Input: part model. Units: mm. Frame: model coordinates. Round coordinates to 2 decimals unless told otherwise and drop trailing zeros. Loops run counter-clockwise (first coordinate to the right, second up) from the corner with the lowest first, then second, coordinate; pieces in that order, holes last.
1) Section A-A, the plane z = -94. Return loops of the section in (x, y), and give its area (3 significant figures).
2) First-contact query: pin 1 (0.9 mm diameter, centred on x = -47, y = 1, fed in from +Z); pin 2 (1.5 mm diameter, centred on x = -105, y = 1, fed in from +Z); pin 3 (0.9 mm diameter, centred on x = -47, y = 1.5, fed in from -Z). Flat tips, straight axial feed; report the tip coordinate or a pass-through.
3) Section B-B, the plane x = -156. Return loops of the section in (y, z), and give its area (3 significant figures).
4) Section C-C, the plane y = 1.85. State how many separate pieces and enclosed holes the cut face has, and give its area (3 significant figures).
5) Section D-D, the plane z = -51. Return loops of the section in (x, y), and give its area (3 significant figures).
6) Ray query, line 1 along Z through (x, y) = (-160, 1.05); line 2 along Z through (x, y) = (-127.5, 1.9); line 3 along X through (y, z) = (2.75, -86.5). Return the intervals inside material, ascending.
Autodesk Inventor part; units mm, degrees
ref_plane "YZ Plane" through (0, 0, 0) normal (1, 0, 0) x (0, 1, 0)
ref_plane "XZ Plane" through (0, 0, 0) normal (0, 1, 0) x (-1, 0, 0)
ref_plane "XY Plane" through (0, 0, 0) normal (0, 0, 1) x (1, 0, 0)
sketch "Sketch1" plane through (0, 0, 0) normal (0, 1, 0) x (-1, 0, 0)
  line L0 (98.8824, -242.8336) -> (78.8824, -242.8336)
  line L1 (98.8824, -237.8336) -> (98.8824, -242.8336)
  line L2 (113.8824, -237.8336) -> (98.8824, -237.8336)
  line L3 (128.8824, -242.8336) -> (113.8824, -242.8336)
  line L4 (128.8824, -242.8336) -> (128.8824, -237.8336)
  line L5 (113.8824, -242.8336) -> (113.8824, -237.8336)
  line L6 (113.8824, 65.1664) -> (113.8824, 62.1664)
  line L7 (98.8824, 62.1664) -> (98.8824, 65.1664)
  line L8 (78.8824, 65.1664) -> (98.8824, 65.1664)
  line L9 (98.8824, 62.1664) -> (113.8824, 62.1664)
  line L10 (113.8824, 65.1664) -> (128.8824, 65.1664)
  line L11 (128.8824, 62.1664) -> (128.8824, 65.1664)
  line L12 (78.8824, 62.1664) -> (78.8824, 65.1664)
  line L13 (63.8824, 62.1664) -> (78.8824, 62.1664)
  line L14 (63.8824, 65.1664) -> (63.8824, 62.1664)
  line L15 (63.8824, -242.8336) -> (63.8824, -237.8336)
  line L16 (63.8824, -237.8336) -> (75.0605, -237.8336)
  line L17 (78.8824, -237.8336) -> (78.8824, -242.8336)
  line L18 (78.8824, -237.8336) -> (63.8824, -237.8336)
  line L19 (63.8824, -237.8336) -> (78.8824, -237.8336)
  line L20 (48.8824, -65.4156) -> (48.8824, -20.7764)
  line L21 (48.8824, -65.4156) -> (48.8824, -20.7764)
  line L22 (48.8824, -65.4156) -> (45.8824, -65.4156)
  line L23 (45.8824, -112.2516) -> (45.8824, -65.4156)
  line L24 (48.8824, -20.7764) -> (45.8824, -20.7764)
  line L25 (48.8824, -202.2369) -> (45.8824, -202.2369)
  line L26 (48.8824, -156.8908) -> (45.8824, -156.8908)
  line L27 (45.8824, -202.2369) -> (45.8824, -156.8908)
  line L28 (48.8824, -112.2516) -> (45.8824, -112.2516)
  line L29 (48.8824, -156.8908) -> (48.8824, -112.2516)
  line L30 (48.8824, -156.8908) -> (48.8824, -112.2516)
  line L31 (45.8824, -20.7764) -> (45.8824, 24.5697)
  line L32 (48.8824, 24.5697) -> (45.8824, 24.5697)
  line L33 (48.8824, 24.5697) -> (48.8824, 62.1664)
  line L34 (48.8824, 65.1664) -> (63.8824, 65.1664)
  line L35 (48.8824, 24.5697) -> (48.8824, 65.1664)
  line L36 (48.8824, -237.8336) -> (48.8824, -202.2369)
  line L37 (48.8824, -242.8336) -> (63.8824, -242.8336)
  line L38 (48.8824, -242.8336) -> (48.8824, -237.8336)
  line L39 (164.8824, -115.3336) -> (164.8824, -112.3336)
  line L40 (164.8824, -112.3336) -> (149.8824, -112.3336)
  line L41 (149.8824, -112.3336) -> (149.8824, -115.3336)
  line L42 (134.8824, -115.3336) -> (134.8824, -112.3336)
  line L43 (134.8824, -112.3336) -> (119.8824, -112.3336)
  line L44 (119.8824, -112.3336) -> (119.8824, -115.3336)
  line L45 (119.8824, -115.3336) -> (134.8824, -115.3336)
  line L46 (149.8824, -115.3336) -> (164.8824, -115.3336)
  line L47 (171.6524, -88.8336) -> (171.6524, -237.8336)
  line L48 (171.6524, -237.8336) -> (128.8824, -237.8336)
  line L49 (171.6524, -88.8336) -> (171.6524, 62.1664)
  line L50 (171.6524, 62.1664) -> (128.8824, 62.1664)
  line L51 (164.8824, -62.3336) -> (164.8824, -65.3336)
  line L52 (164.8824, -65.3336) -> (149.8824, -65.3336)
  line L53 (149.8824, -65.3336) -> (149.8824, -62.3336)
  line L54 (134.8824, -62.3336) -> (134.8824, -65.3336)
  line L55 (134.8824, -65.3336) -> (119.8824, -65.3336)
  line L56 (119.8824, -65.3336) -> (119.8824, -62.3336)
  line L57 (119.8824, -62.3336) -> (134.8824, -62.3336)
  line L58 (149.8824, -62.3336) -> (164.8824, -62.3336)
  line L59 (76.2158, -102.1043) -> (81.5491, -102.1043)
  line L60 (83.5491, -100.1043) -> (83.5491, -77.5629)
  line L61 (81.5491, -75.5629) -> (76.2158, -75.5629)
  line L62 (74.2158, -77.5629) -> (74.2158, -100.1043)
  line L63 (74.2158, -102.1043) -> (83.5491, -75.5629) construction
  line L64 (83.5491, -102.1043) -> (74.2158, -75.5629) construction
  arc A0 (83.5491, -77.5629) -> (81.5491, -75.5629) centre (81.5491, -77.5629) ccw
  arc A1 (76.2158, -75.5629) -> (74.2158, -77.5629) centre (76.2158, -77.5629) ccw
  arc A2 (81.5491, -102.1043) -> (83.5491, -100.1043) centre (81.5491, -100.1043) ccw
  arc A3 (74.2158, -100.1043) -> (76.2158, -102.1043) centre (76.2158, -100.1043) ccw
  point P0 (0, 0)
  point P1 (0, 0)
  point P2 (106.3824, -237.8336)
  point P3 (106.3824, 62.1664)
  point P4 (121.3824, 65.1664)
  point P5 (47.3824, -202.2369)
  point P6 (78.8824, -88.8336)
  dimension "d0" = 80
  dimension "d1" = 15
  dimension "d2" = 15
  dimension "d3" = 300
  dimension "d5" = 3
  dimension "d6" = 5
  dimension "d7" = 44.6392
  dimension "d8" = 37.5967
  dimension "d9" = 44.6392
  dimension "d10" = 40.5967
  dimension "d11" = 45.3461
  dimension "d12" = 46.8359
  dimension "d13" = 45.3461
  dimension "d14" = 20
  dimension "d15" = 15
  dimension "d16" = 15
  dimension "d17" = 15
  dimension "d18" = 15
  dimension "d19" = 15
  dimension "d20" = 15
  dimension "d21" = 20
  dimension "d22" = 308
  dimension "d29" = 3
  dimension "d30" = 15
  dimension "d31" = 3
  dimension "d32" = 15
  dimension "d33" = 3
  dimension "d34" = 15
  dimension "d38" = 2
extrude "Extrusion1" add sketch "Sketch1" along normal blind 3
properties part number "mieng_ben_gan_sensor_3mm"
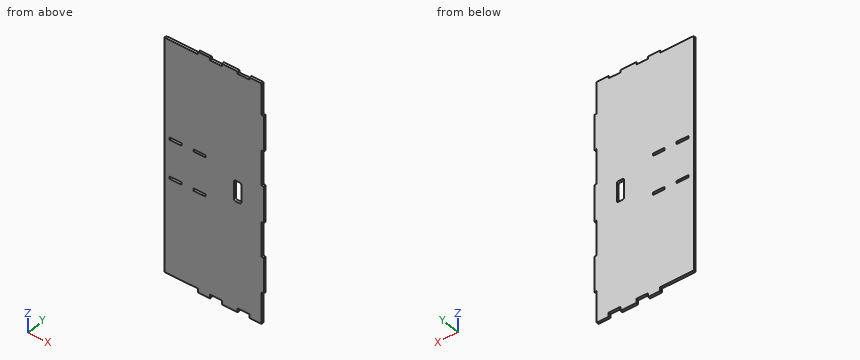
Final values:
1. outline: (-171.65, 0) - (-83.55, 0) - (-83.55, 3) - (-171.65, 3) - close; (-74.22, 0) - (-45.88, 0) - (-45.88, 3) - (-74.22, 3) - close
1. area: 349 mm2
2. pin 1: stops at z = 24.57
2. pin 2: stops at z = 62.17
2. pin 3: stops at z = -202.24
3. outline: (0, -237.83) - (3, -237.83) - (3, -115.33) - (0, -115.33) - close; (0, -112.33) - (3, -112.33) - (3, -65.33) - (0, -65.33) - close; (0, -62.33) - (3, -62.33) - (3, 62.17) - (0, 62.17) - close
3. area: 882 mm2
4. separate pieces: 1
4. enclosed holes: 5
4. area: 37,200 mm2
5. outline: (-171.65, 0) - (-48.88, 0) - (-48.88, 3) - (-171.65, 3) - close
5. area: 368 mm2
6. line 1: z = -237.83 to -115.33, -112.33 to -65.33, -62.33 to 62.17
6. line 2: z = -242.83 to -115.33, -112.33 to -65.33, -62.33 to 65.17
6. line 3: x = -171.65 to -83.55, -74.22 to -45.88
